```python
from build123d import *

# Parameters (mm, degrees)
SKETCH1_W           = 1000
SKETCH1_H           = 30
BOSS_EXTRUDE1_DEPTH = 350
SKETCH2_W           = 1000
SKETCH2_H           = 30
SKETCH2_H_2         = 5
BOSS_EXTRUDE2_DEPTH = 30
LPATTERN1_COUNT     = 2
LPATTERN1_PITCH     = 380
SKETCH3_R           = 5
CUT_EXTRUDE1_DEPTH  = 1100.874992897


with BuildPart() as part:
    # Sketch1 → Boss-Extrude1 (new body)
    with BuildSketch(Plane(origin=(0, 0, 0), x_dir=(0, 0, -1), z_dir=(1, 0, 0))):
        with BuildLine():
            Line((0, 0), (0, 30))
            ThreePointArc((0, 30), (-15, 15), (0, 0))
        make_face()
        with Locations((500, 15)):
            Rectangle(SKETCH1_W, SKETCH1_H)
        with BuildLine():
            ThreePointArc((1000, 30), (1015, 15), (1000, 0))
            Line((1000, 0), (1000, 30))
        make_face()
    extrude(amount=BOSS_EXTRUDE1_DEPTH)

    # Sketch2 → Boss-Extrude2 (add)
    with BuildSketch(Plane(origin=(350, 0, 0), x_dir=(0, 0, -1), z_dir=(1, 0, 0))):
        with BuildLine():
            ThreePointArc((0, 35), (-20, 15), (0, -5))
            Line((0, -5), (0, 0))
            ThreePointArc((0, 0), (-15, 15), (0, 30))
            Line((0, 30), (0, 35))
        make_face()
        with BuildLine():
            ThreePointArc((0, 30), (-15, 15), (0, 0))
            Line((0, 0), (0, 30))
        make_face()
        with Locations((500, 15)):
            Rectangle(SKETCH2_W, SKETCH2_H)
        with Locations((500, 32.5)):
            Rectangle(SKETCH2_W, SKETCH2_H_2)
        with Locations((500, -2.5)):
            Rectangle(SKETCH2_W, SKETCH2_H_2)
        with BuildLine():
            Line((1000, 30), (1000, 0))
            ThreePointArc((1000, 0), (1015, 15), (1000, 30))
        make_face()
        with BuildLine():
            Line((1000, 0), (1000, -5))
            ThreePointArc((1000, -5), (1020, 15), (1000, 35))
            Line((1000, 35), (1000, 30))
            ThreePointArc((1000, 30), (1015, 15), (1000, 0))
        make_face()
    boss_extrude2 = extrude(amount=BOSS_EXTRUDE2_DEPTH)

    # LPattern1: Boss-Extrude2 ×2
    with Locations(*[(-i * LPATTERN1_PITCH, 0, 0) for i in range(1, LPATTERN1_COUNT)]):
        add(boss_extrude2)

    # Sketch3 → Cut-Extrude1 (cut, through all)
    with BuildSketch(Plane(origin=(380, 0, 0), x_dir=(0, 0, -1), z_dir=(1, 0, 0))):
        with Locations((0, 15)):
            Circle(SKETCH3_R)
        with Locations((1000, 15)):
            Circle(SKETCH3_R)
    extrude(amount=-CUT_EXTRUDE1_DEPTH, mode=Mode.SUBTRACT)


solid = part.part
```
For this review, take the finished solid that the model builds, in its own axes (mm). A direction names the side the tool comes from. Round coordinates to 2 decimals unless told otherwise and drop trailing zeros. Write each loop counter-clockwise with the first axis right and the second up, starting at its lowest first coordinate (ties: lowest second). Pieces come first, ordered by that corner, then holes. Notation, with made-up numbers: (51, 88) - (65, 88) arc R19 ccw to (65, 98) - close; hole circle Ø5 at (33.25, 63.5). An arc over 180 degrees is marked (long way). Write each question's results on one line, items separated by ' | '.
Item 1: Take a section at A-A on z = -502.5. State the section outline as (x, y) points.
Calculated:
outline: (-30, -5) - (0, -5) - (0, 0) - (350, 0) - (350, -5) - (380, -5) - (380, 35) - (350, 35) - (350, 30) - (0, 30) - (0, 35) - (-30, 35) - close
Item 2: Draft analysis for pull direction X (two halves, no side actions). For faces 4 (the face through (-15, 15, -1020)), 5 (the face through (173, 15, -1015)), 6 (the face through (380, 15, -493)), state which applies: pulls with the +X half, pulls with the -X half, needs draft (parallel to the pull), parting line crosses it, or undercut.
Calculated:
face 4: needs draft | face 5: undercut | face 6: pulls with the +X half
Item 3: To check wall thickness, follow line 1 along X through (y, z) = (-3, -213.5); line 2 along Z through (x, y) = (343.5, 19); line 3 along Y through (x, z) = (102.5, -1000). State the ranges of each line that lie inside material, in increasing order. Write a range as from..to.
Calculated:
line 1: x = -30..0, 350..380 | line 2: z = -1014.46..-1003, -997..-3, 3..14.46 | line 3: y = 0..10, 20..30
Item 4: For pin 1 (13 mm diameter, centred on y = 15, z = 0, fed in from +X); pin 2 (5 mm diameter, centred on x = 55, y = 0, fed in from -Z); pin 3 (3 mm diameter, centred on x = 88.5, y = 16.5, fed in from -Z); pin 4 (3 mm diameter, centred on x = 97, z = -610.5, fed in from -Y), all flat-tipped, find the tip position at first contact; note any pin that passes through.
Calculated:
pin 1: stops at x = 380 | pin 2: stops at z = -1008.29 | pin 3: stops at z = -1015 | pin 4: stops at y = 0
Item 5: Take a section at B-B on x = 137.5. State the section outline as (y, z) points.
Calculated:
outline: (0, -1000) arc R15 ccw to (30, -1000) - (30, 0) arc R15 ccw to (0, 0) - close; hole circle Ø10 at (15, -1000); hole circle Ø10 at (15, 0)
Item 6: For faces 1 (the face through (173, 15, 15)), 2 (the face through (173, 0, -493)), 3 (the face through (173, 30, -493)), list the 3-axis set-ups (+Z, -Z, +X, -X, +Y, -Y) from which the entire face can be reached by the end or side of a thin tool; tool diameter is ignored.
Calculated:
face 1: +Z | face 2: +Z, -Z, -Y | face 3: +Z, -Z, +Y
